Design review of the part shown in the three views and the two pictorial views. Dimensions are in mm from the part's minimum x, y and z. Round coordinates to 2 decimals unless told otherwise and drop trailing zeros. Return JSON: item names as keys, results as strings. Group by question number.
(1) Wall thickness on L1, parallel to X at y = 24.5, z = 4.5 (1 decimal); L2, parallel to X at y = 26.5, z = 2.5 (1 decimal); L3, parallel to Y at x = 310, z = 4.5: over which ranges is each line inside the solid? List them lowest first. Write a range as [from, to].
(2) We need section A-A, the plane y = 25.4. Give the number of separate pieces and of enclosed holes in the cut face, and give its area (3 significant figures).
(3) Clearance check with a flat-ended pin moving along its axis: pin 1 (3 mm diameter, centred on y = 8, z = 5, fed in from -X) (1 decimal). State where the tip first meets the part, or that it passes through.
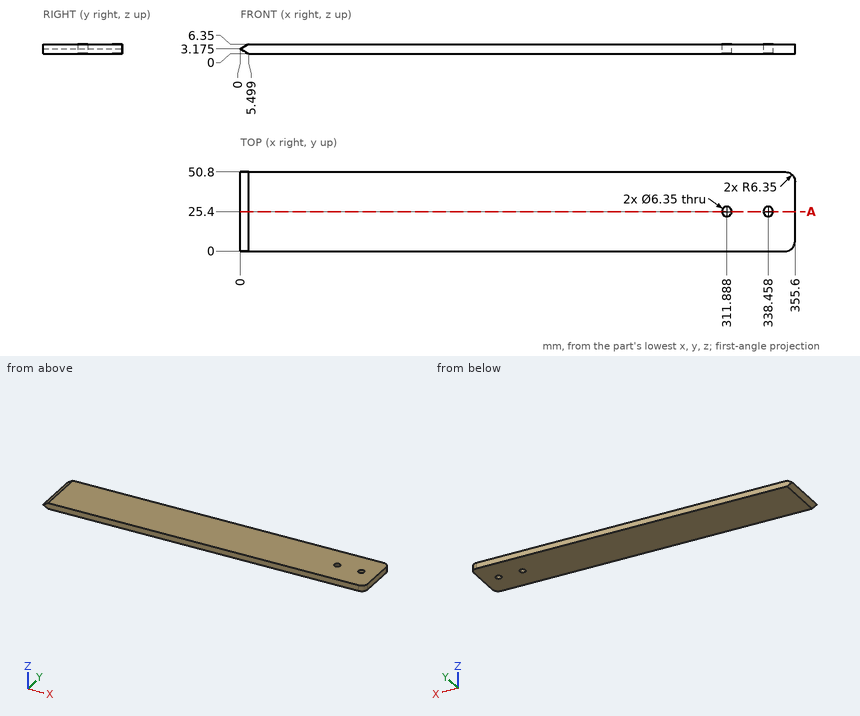
Solutions:
{
 "1": {"L1": "[2.3, 308.8], [314.9, 335.4], [341.5, 355.6]", "L2": "[1.2, 308.9], [314.9, 335.5], [341.4, 355.6]", "L3": "[0, 22.85], [27.95, 50.8]"},
 "2": {"separate pieces": "3", "enclosed holes": "0", "area": "2,160 mm^2"},
 "3": {"pin 1": "x = 0.6"}
}
